Can you work these out from the drawing? Everything is in mm from the part's minimum corner. A direction names the side the tool comes from. Round coordinates to 2 decimals unless told otherwise and drop trailing zeros. Loops run counter-clockwise (first coordinate to the right, second up) from the corner with the lowest first, then second, coordinate; pieces in that order, holes last. Notation, with made-up numbers: (1, 27) - (40, 27) arc R22 ccw to (40, 41) - close; hole circle Ø5 at (87, 13). An arc over 180 degrees is marked (long way). Answer as a JSON object with one key per item and string values. Group by question number.
1) If I drill on line 1 along Z through (x, y) = (3.25, 18.25); line 2 along X through (y, z) = (15.25, 82.5); line 3 along Z through (x, y) = (15, 22), over which ranges is the centre line in solid material (lowest first)? Write a range as [from, to].
2) I want a section at C-C, the plane z = 48. Please give me the cut outline in (x, y), then the cut area to 3 significant figures.
3) Will these pins go through, and if not, where does the flat tip stop? P1, Ø6, axis at y = 8.5, z = 64.5, coming from the -X side; P2, Ø4, axis at x = 24.5, z = 97.5, coming from the -Y side; P3, Ø5, axis at x = 16, z = 5, coming from the +Y side.
4) I want a section at A-A, the plane x = 15. Please give me the cut outline in (y, z).
5) I want a section at B-B, the plane y = 15. Please give me the cut outline in (x, z).
6) I want a section at D-D, the plane x = 2.75. Please give me the cut outline in (y, z), then the cut area to 3 significant figures.
7) Which directions (+Z, -Z, +X, -X, +Y, -Y) give clear straight access to the entire face, cutting with the end or side of a thin tool? Please do the marked faces 1, 2 and 3.
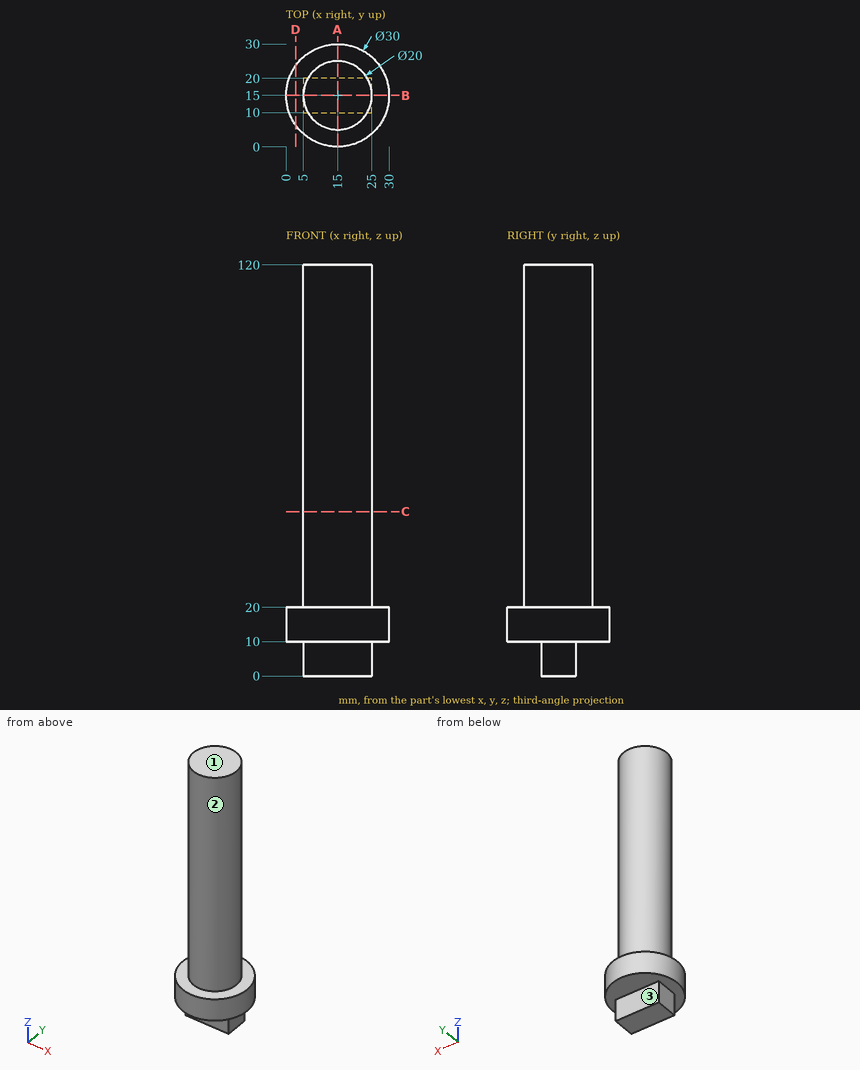
Outcome:
{
 "1": {"line 1": "[10, 20]", "line 2": "[5, 25]", "line 3": "[10, 120]"},
 "2": {"outline": "circle Ø20 at (15, 15)", "area": "314 mm^2"},
 "3": {"P1": "x = 5.63", "P2": "y = 8.39", "P3": "y = 20"},
 "4": {"outline": "(0, 10) - (10, 10) - (10, 0) - (20, 0) - (20, 10) - (30, 10) - (30, 20) - (25, 20) - (25, 120) - (5, 120) - (5, 20) - (0, 20) - close"},
 "5": {"outline": "(0, 10) - (5, 10) - (5, 0) - (25, 0) - (25, 10) - (30, 10) - (30, 20) - (25, 20) - (25, 120) - (5, 120) - (5, 20) - (0, 20) - close"},
 "6": {"outline": "(6.34, 10) - (23.66, 10) - (23.66, 20) - (6.34, 20) - close", "area": "173 mm^2"},
 "7": {"face 1": "+Z, +X, -X, +Y, -Y", "face 2": "+Z", "face 3": "-Z, +X, -X, +Y"}
}
